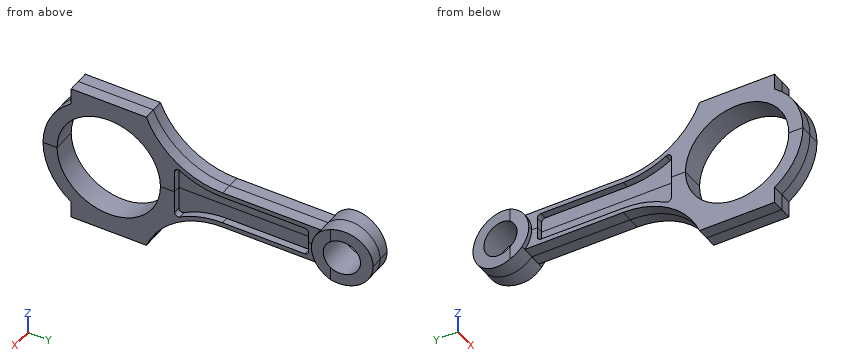
from build123d import *
from build123d import SkipClean  # not in build123d's __all__

# Parameters (mm, degrees)
F1_DEPTH = 7
F2_DEPTH = 5
F3_DEPTH = 2
F7_DEPTH = 25


with BuildPart() as f1:
    # F0 (on Right) → F1 (new body)
    with BuildSketch(Plane.YZ):
        with BuildLine():
            ThreePointArc((107.5, 0), (100, -7.5), (92.5, 0))
            Line((92.5, 0), (87.5, 0))
            ThreePointArc((87.5, 0), (88.2460947032, -4.2539052968), (90.3953136439, -8))
            ThreePointArc((90.3953136439, -8), (104.2539052968, -11.7539052968), (112.5, 0))
            Line((112.5, 0), (107.5, 0))
        make_face()
    extrude(amount=F1_DEPTH)

    # F0 (on Right) → F2 (join)
    with BuildSketch(Plane.YZ):
        with BuildLine():
            ThreePointArc((90.3953136439, -8), (88.2460947032, -4.2539052968), (87.5, 0))
            Line((87.5, 0), (85, 0))
            Line((85, 0), (85, -4.5))
            ThreePointArc((85, -4.5), (84.5606601718, -5.5606601718), (83.5, -6))
            Line((83.5, -6), (48.4961536185, -6))
            ThreePointArc((48.4961536185, -6), (39.0556702336, -7.2246275567), (30.2401098812, -10.8174446779))
            ThreePointArc((30.2401098812, -10.8174446779), (28.7450711364, -10.8089264191), (28, -9.5127464891))
            Line((28, -9.5127464891), (28, 0))
            Line((28, 0), (22, 0))
            ThreePointArc((22, 0), (0, -22), (-22, 0))
            Line((-22, 0), (-28, 0))
            ThreePointArc((-28, 0), (-24.819347292, -12.9614813968), (-16, -22.9782505862))
            Line((-16, -22.9782505862), (-16, -30))
            Line((-16, -30), (16, -30))
            ThreePointArc((16, -30), (28.8747367482, -14.0172465076), (48.4961536185, -8))
            Line((48.4961536185, -8), (90.3953136439, -8))
        make_face()
    extrude(amount=F2_DEPTH)

    # F0 (on Right) → F3 (join)
    with BuildSketch(Plane.YZ):
        with BuildLine():
            Line((85, -4.5), (85, 0))
            Line((85, 0), (28, 0))
            Line((28, 0), (28, -9.5127464891))
            ThreePointArc((28, -9.5127464891), (28.7450711364, -10.8089264191), (30.2401098812, -10.8174446779))
            ThreePointArc((30.2401098812, -10.8174446779), (39.0556702336, -7.2246275567), (48.4961536185, -6))
            Line((48.4961536185, -6), (83.5, -6))
            ThreePointArc((83.5, -6), (84.5606601718, -5.5606601718), (85, -4.5))
        make_face()
    extrude(amount=F3_DEPTH)

    # F4: F1 across plane


with BuildPart() as f1_1:
    add(f1.part, clean=False)
    add(f1.part.mirror(Plane.YZ), clean=False)

    # F5: F1 across plane


with BuildPart() as f1_2:
    add(f1_1.part, clean=False)
    with SkipClean():  # cleaning this boolean's faces spoils the solid; the shape is the same uncleaned
        add(f1_1.part.mirror(Plane.XY), clean=False)

    # F6 (on Top) → F7 (cut, symmetric)
    with BuildSketch(Plane.XY):
        Polygon((-7, 112.5), (-7, 95.5), (-4.9126624647, 112.5), align=None)
        Polygon((4.9126624647, 112.5), (7, 95.5), (7, 112.5), align=None)
    with SkipClean():  # cleaning this boolean's faces spoils the solid; the shape is the same uncleaned
        extrude(amount=F7_DEPTH, both=True, mode=Mode.SUBTRACT)


solid = f1_2.part
The model under review builds one solid part; all positions refer to its coordinate system, in mm. Coordinates: 2 decimals unless noted, no trailing zeros. Write each loop counter-clockwise with the first axis right and the second up, starting at its lowest first coordinate (ties: lowest second). Pieces come first, ordered by that corner, then holes. Notation, with made-up numbers: (4, 13) - (48, 13) arc R32 cw to (48, 46) - close; hole circle Ø7 at (-16.5, 75). An arc over 180 degrees is marked (long way). Answer as CSV lines item,"result".
(1) Clearance check with flat-ended pins moving along their axes: pin 1 Ø1.5 at (x, z) = (3.5, -26.5) entering from -Y; pin 2 Ø12 at (y, z) = (52, -5.5) entering from +X; pin 3 Ø13.5 at (y, z) = (100, 0) entering from -X; pin 4 Ø1 at (x, y) = (1, 32.5) entering from -Z. State where each tip first meets the part, or that it passes through.
Data:
pin 1,"stops at y = -16"
pin 2,"stops at x = 5"
pin 3,"passes through"
pin 4,"stops at z = -12.13"
(2) For line 1 along Y through (x, z) = (-4, 0); line 2 along Z through (x, y) = (3.25, 68); line 3 along Z through (x, y) = (0, 100), list the stretches that pass through material, from the lowest coordinate up. Write a range as [from, to].
Data:
line 1,"y = [-28, -22], [22, 28], [85, 92.5], [107.5, 112.5]"
line 2,"z = [-8, -6], [6, 8]"
line 3,"z = [-12.5, -7.5], [7.5, 12.5]"
(3) We need section A-A (y = 0). Give the boundary of the cut face in (x, z), plus the area to 3 significant figures.
Data:
outline,"(-5, -30) - (5, -30) - (5, -22) - (-5, -22) - close; (-5, 22) - (5, 22) - (5, 30) - (-5, 30) - close"
area,"160 mm2"
(4) We need section D-D (z = -2.5). Give the boundary of the cut face in (x, y).
Data:
outline,"(-7, 87.75) - (-5, 87.75) - (-5, 85) - (-2, 85) - (-2, 28) - (-5, 28) - (-5, 21.86) - (5, 21.86) - (5, 28) - (2, 28) - (2, 85) - (5, 85) - (5, 87.75) - (7, 87.75) - (7, 92.93) - (-7, 92.93) - close; (-5.58, 107.07) - (5.58, 107.07) - (4.94, 112.25) - (-4.94, 112.25) - close; (-5, -27.89) - (5, -27.89) - (5, -21.86) - (-5, -21.86) - close"
(5) We need section B-B (x = 3.5). Give the boundary of the cut face in (y, z).
Data:
outline,"(-16, -30) - (16, -30) arc R35 cw to (48.5, -8) - (90.4, -8) arc R12.5 ccw (long way) to (90.4, 8) - (48.5, 8) arc R35 cw to (16, 30) - (-16, 30) - (-16, 22.98) arc R28 ccw to (-16, -22.98) - close; hole circle Ø44 at (0, 0); hole (28, -9.51) arc R1.5 ccw to (30.24, -10.82) arc R37 cw to (48.5, -6) - (83.5, -6) arc R1.5 ccw to (85, -4.5) - (85, 4.5) arc R1.5 ccw to (83.5, 6) - (48.5, 6) arc R37 cw to (30.24, 10.82) arc R1.5 ccw to (28, 9.51) - close; hole circle Ø15 at (100, 0)"
(6) We need section C-C (z = 18.5). Give the boundary of the cut face in (x, y).
Data:
outline,"(-5, -21.02) - (5, -21.02) - (5, -11.91) - (-5, -11.91) - close; (-5, 11.91) - (5, 11.91) - (5, 23.5) - (-5, 23.5) - close"
